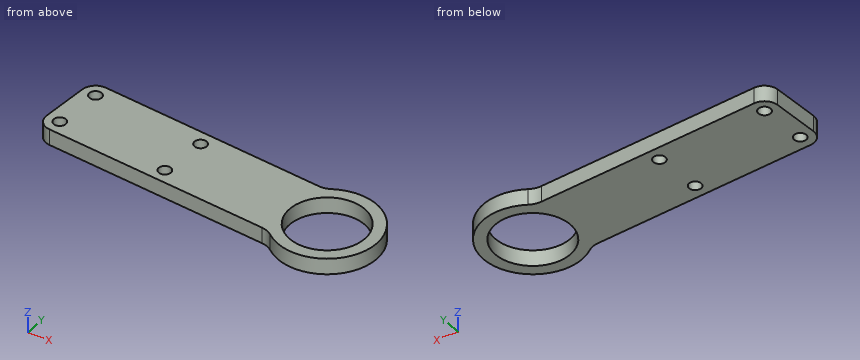
```python
from build123d import *

# Parameters (mm, degrees)
SKETCH_1_R          = 6
EXTRUDE_1_DEPTH     = 2
SKETCH_2_R          = 1.55
SKETCH_2_R_2        = 0.6
CUT_EXTRUDE_1_DEPTH = 5
FILLET_1_R          = 3.5
SKETCH_3_OUTSIDE_W  = 217.41
SKETCH_3_OUTSIDE_H  = 71.355
CUT_EXTRUDE_2_DEPTH = 5
SKETCH_4_R          = 1.55
CUT_EXTRUDE_3_DEPTH = 5
FILLET_2_R          = 3.5
SKETCH_5_R          = 12.5
EXTRUDE_2_DEPTH     = 4
SKETCH_6_R          = 9.5
CUT_EXTRUDE_4_DEPTH = 5
FILLET_3_R          = 5


with BuildPart() as part:
    # 草图1 → 凸台-拉伸1 (new body, symmetric)
    with BuildSketch(Plane.XY):
        with BuildLine():
            Line((-8.927079897, 3.249191362), (-1.4961968, 23.665374879))
            Line((-1.4961968, 23.665374879), (160.827979556, 9.463849632))
            ThreePointArc((160.827979556, 9.463849632), (169.463849632, -0.827979556), (159.172020444, -9.463849632))
            Line((159.172020444, -9.463849632), (11.371578553, 3.467013498))
            Line((11.371578553, 3.467013498), (8.927079897, -3.249191362))
            ThreePointArc((8.927079897, -3.249191362), (-3.249191362, -8.927079897), (-8.927079897, 3.249191362))
        make_face()
        Circle(SKETCH_1_R, mode=Mode.SUBTRACT)
        with Locations((160, 0)):
            Circle(SKETCH_1_R, mode=Mode.SUBTRACT)
    extrude(amount=EXTRUDE_1_DEPTH, both=True)

    # 草图2 → 切除-拉伸1 (cut, through all)
    with BuildSketch(Plane.XY.offset(2)):
        with Locations((0.874182871, 19.944624098)):
            Circle(SKETCH_2_R)
        with Locations((16.220555377, 6.556152427)):
            Circle(SKETCH_2_R)
        with Locations((11.935394126, 3.261801412)):
            Circle(SKETCH_2_R_2)
    extrude(amount=-CUT_EXTRUDE_1_DEPTH, mode=Mode.SUBTRACT)

    # 圆角1
    fillet_1_edges = [part.edges().sort_by_distance(p)[0] for p in [
        (-1.4961968, 23.665374879, 0),
    ]]
    fillet(fillet_1_edges, radius=FILLET_1_R)

    # 草图3 outside → 切除-拉伸2 (cut, through all)
    with BuildSketch(Plane.XY.offset(2)):
        with Locations((80, 6.9725)):
            Rectangle(SKETCH_3_OUTSIDE_W, SKETCH_3_OUTSIDE_H)
        with BuildLine():
            Line((91.09435069, 15.564751624), (89.438391577, -3.36294764))
            Line((89.438391577, -3.36294764), (159.172020444, -9.463849632))
            ThreePointArc((159.172020444, -9.463849632), (169.463849632, -0.827979556), (160.827979556, 9.463849632))
            Line((160.827979556, 9.463849632), (91.09435069, 15.564751624))
        make_face(mode=Mode.SUBTRACT)
    extrude(amount=-CUT_EXTRUDE_2_DEPTH, mode=Mode.SUBTRACT)

    # 草图4 → 切除-拉伸3 (cut, through all)
    with BuildSketch(Plane.XY.offset(2)):
        with Locations((94.275987033, 11.773025081)):
            Circle(SKETCH_4_R)
        with Locations((93.23011812, -0.181311296)):
            Circle(SKETCH_4_R)
        with Locations((122.16943858, 9.332664284)):
            Circle(SKETCH_4_R)
        with Locations((121.123569667, -2.621672093)):
            Circle(SKETCH_4_R)
    extrude(amount=-CUT_EXTRUDE_3_DEPTH, mode=Mode.SUBTRACT)

    # 圆角2
    fillet_2_edges = [part.edges().sort_by_distance(p)[0] for p in [
        (89.438391577, -3.36294764, 0),
        (91.09435069, 15.564751624, 0),
    ]]
    fillet(fillet_2_edges, radius=FILLET_2_R)

    # 草图5 → 凸台-拉伸2 (add)
    with BuildSketch(Plane.XY.offset(2)):
        with Locations((160, 0)):
            Circle(SKETCH_5_R)
    extrude(amount=-EXTRUDE_2_DEPTH)

    # 草图6 → 切除-拉伸4 (cut, through all)
    with BuildSketch(Plane.XY.offset(2)):
        with Locations((160, 0)):
            Circle(SKETCH_6_R)
    extrude(amount=-CUT_EXTRUDE_4_DEPTH, mode=Mode.SUBTRACT)

    # 圆角3
    fillet_3_edges = [part.edges().sort_by_distance(p)[0] for p in [
        (152.73485557, 10.171906233, 0),
        (151.078896458, -8.755793031, 0),
    ]]
    fillet(fillet_3_edges, radius=FILLET_3_R)


solid = part.part
```
Source: CAD feature listing. Evaluate the final solid. Frame: model axes, mm. Give positions to 0.01 mm unless a question says otherwise; leave off trailing zeros. Order: outer loops, then holes, each group sorted by start corner. A loop starts at its lowest first (then second) coordinate and runs counter-clockwise, first axis right, second up.
(1) Section query C-C (z = -0.4). Return the cut outline in (x, y).
(2) Material intervals for line 1 along Y through (x, z) = (122.5, 1.8); line 2 along X through (y, z) = (-2.5, 0.1); line 3 along Y through (x, z) = (95, -0.65), sorted ascending.
(3) Section query A-A (x = 160). Return the cut outline in (y, z).
(4) Section query B-B (y = 6.5). Return the cut outline in (x, z).
(5) Section query D-D (x = 125). Return the cut outline in (y, z).
(6) Contact query for flat-ended pins moving along their axis: P1, Ø3.5, axis at x = 121.12, y = -2.62, coming from the +Z side; P2, Ø1.5, axis at y = 11, z = 1, coming from the -X side; P3, Ø2, axis at x = 146, z = 0.5, coming from the -Y side. Output: stop coordinate, or through.
Outcome:
1. outline: (89.74, 0.12) arc R3.5 ccw to (92.93, -3.67) - (149.41, -8.61) arc R5 cw to (152.13, -9.71) arc R12.5 ccw (long way) to (153.93, 10.93) arc R5 cw to (151.07, 10.32) - (94.58, 15.26) arc R3.5 ccw to (90.79, 12.08) - close; hole circle Ø3.1 at (93.23, -0.18); hole circle Ø3.1 at (94.28, 11.77); hole circle Ø3.1 at (121.12, -2.62); hole circle Ø3.1 at (122.17, 9.33); hole circle Ø19 at (160, 0)
2. line 1: y = -6.26 to -3.33, -1.91 to 7.82, 10.85 to 12.82
2. line 2: x = 90.61 to 119.58, 122.67 to 150.83, 169.17 to 172.25
2. line 3: y = -3.85 to 10.4, 13.14 to 15.22
3. outline: (-12.5, -2) - (-9.5, -2) - (-9.5, 2) - (-12.5, 2) - close; (9.5, -2) - (12.5, -2) - (12.5, 2) - (9.5, 2) - close
4. outline: (90.3, -2) - (153.07, -2) - (153.07, 2) - (90.3, 2) - close; (166.93, -2) - (170.68, -2) - (170.68, 2) - (166.93, 2) - close
5. outline: (-6.47, -2) - (12.6, -2) - (12.6, 2) - (-6.47, 2) - close
6. P1: stops at z = 2
6. P2: stops at x = 90.63
6. P3: stops at y = -8.4
